```python
from build123d import *

# Parameters (mm, degrees)
F0_R     = 25
F0_R_2   = 12.5
F3_DEPTH = 50
F1_W     = 50
F1_H     = 19.626164
F1_R     = 5.973153
F4_DEPTH = 25
F2_R     = 25
F2_R_2   = 2.5
F5_DEPTH = 25


with BuildPart() as f3:
    # F0 (on Top) → F3 (new body)
    with BuildSketch(Plane.XY):
        Circle(F0_R)
        Circle(F0_R_2, mode=Mode.SUBTRACT)
    extrude(amount=F3_DEPTH)


with BuildPart() as f4:
    # F1 (on Right) → F4 (new body, symmetric)
    with BuildSketch(Plane.YZ):
        with Locations((0, 9.813082)):
            Rectangle(F1_W, F1_H)
        with Locations((0, 10.210484)):
            Circle(F1_R, mode=Mode.SUBTRACT)
    extrude(amount=F4_DEPTH, both=True)


with BuildPart() as f5:
    # F2 (on Front) → F5 (new body, symmetric)
    with BuildSketch(Plane.XZ):
        Circle(F2_R)
        with Locations((0, 10.25444)):
            Circle(F2_R_2, mode=Mode.SUBTRACT)
    extrude(amount=F5_DEPTH, both=True)


with BuildPart() as f3_1:
    add(f3.part)

    # F6: intersect F4, F5
    add(f4.part, mode=Mode.INTERSECT)
    add(f5.part, mode=Mode.INTERSECT)


solid = f3_1.part
```
Geometry check sheet. Reference: the model listing, model coordinates, mm. Give positions to 0.01 mm unless a question says otherwise; leave off trailing zeros. Order: outer loops, then holes, each group sorted by start corner. A loop starts at its lowest first (then second) coordinate and runs counter-clockwise, first axis right, second up. Notation, with made-up numbers: (28.5, -20.5) - (72.5, -20.5) arc R22 ccw to (72.5, -3.5) - close; hole circle Ø5 at (20, 78.5). An arc over 180 degrees is marked (long way). Write item = value, one per line. Start each with the question number.
1) Section check D-D (y = 7.5). Enter the section's corners in (x, z), then the cut area to 3 significant figures.
2) Section check C-C (z = 6.5). Enter the section's corners in (x, y).
3) Section check A-A (x = 0). Enter the section's corners in (y, z).
4) Section check B-B (y = -3.5). Enter the section's corners in (x, z), then the cut area to 3 significant figures.
5) Scan lines: L1, parallel to Y at x = 14, z = 13.75; L2, parallel to Z at x = 0, y = 17; L3, parallel to X at y = -22, z = 10. Record each from-to range of solid material in increasing order.
6) Draft check along Z on faces 1 (the flat face through (-11.5, 5.9, 0)), 2 (the flat face through (-7, 11, 19.626)), 3 (the cylindrical face through (-17.9, -1.29, 4.38)). Enter one of: released by +Z, released by -Z, zero draft, split by the parting line, or undercut.
7) Gauge pin test, flat ends, axial feed: pin 1 Ø10 at (x, z) = (5.5, 13) entering from +Y (3 decimals); pin 2 Ø2 at (x, z) = (17, 6.5) entering from -Y; pin 3 Ø8 at (x, z) = (14, 5.5) entering from +Y. Record the tip position at first contact, or that the pin passes through.
Geometry check:
q1.outline = (-23.85, 0) - (-10, 0) - (-10, 19.63) - (-15.49, 19.63) arc R25 ccw to (-23.85, 7.5) - close; (10, 0) - (23.85, 0) - (23.85, 7.5) arc R25 ccw to (15.49, 19.63) - (10, 19.63) - close
q1.area = 464 mm2
q2.outline = (-24.14, -6.5) arc R25 ccw to (24.14, -6.5) - (24.14, -4.68) - (11.59, -4.68) arc R12.5 cw to (-11.59, -4.68) - (-24.14, -4.68) - close; (-24.14, 4.68) - (-11.59, 4.68) arc R12.5 cw to (11.59, 4.68) - (24.14, 4.68) - (24.14, 6.5) arc R25 ccw to (-24.14, 6.5) - close
q3.outline = (-25, 0) - (-12.5, 0) - (-12.5, 7.75) - (-25, 7.75) - close; (-25, 12.75) - (-12.5, 12.75) - (-12.5, 19.63) - (-25, 19.63) - close; (12.5, 0) - (25, 0) - (25, 7.75) - (12.5, 7.75) - close; (12.5, 12.75) - (25, 12.75) - (25, 19.63) - (12.5, 19.63) - close
q4.outline = (-24.75, 0) - (-12, 0) - (-12, 5.37) - (-24.42, 5.37) arc R25 ccw to (-24.75, 3.5) - close; (-19.96, 15.05) - (-12, 15.05) - (-12, 19.63) - (-15.49, 19.63) arc R25 ccw to start; (12, 0) - (24.75, 0) - (24.75, 3.5) arc R25 ccw to (24.42, 5.37) - (12, 5.37) - close; (12, 15.05) - (19.96, 15.05) arc R25 ccw to (15.49, 19.63) - (12, 19.63) - close
q4.area = 191 mm2
q5.L1 = -20.71 to -4.81, 4.81 to 20.71
q5.L2 = 0 to 7.75, 12.75 to 19.63
q5.L3 = -11.87 to -2.49, 2.49 to 11.87
q6.face_1 = released by -Z
q6.face_2 = released by +Z
q6.face_3 = undercut
q7.pin_1 = 24.995
q7.pin_2 = -19.21
q7.pin_3 = 22.91
